Build history of the part. All positions in model axes, mm. A direction names the side the tool comes from. Coordinates: 2 decimals unless noted, no trailing zeros. Order: outer loops, then holes, each group sorted by start corner. A loop starts at its lowest first (then second) coordinate and runs counter-clockwise, first axis right, second up. Notation, with made-up numbers: M 12,-8 L 60,-8 A32 ccw 60,29 Z; hole C 24.25,49.5 d9. An arc over 180 degrees is marked long. Use a Markdown table: item, result. Add a question column.
from build123d import *

# Parameters (mm, degrees)
ESQUISSE1_W      = 187
ESQUISSE1_H      = 15
ESQUISSE1_R      = 1.5
EXTRUSION1_DEPTH = 1.5
ESQUISSE3_W      = 187
ESQUISSE3_H      = 1.5
EXTRUSION3_DEPTH = 13.5
ESQUISSE4_R      = 1.5
EXTRUSION4_DEPTH = 10


with BuildPart() as part:
    # Esquisse1 → Extrusion1 (new body)
    with BuildSketch(Plane.XY):
        with Locations((13.570945199, 9.544736842)):
            Rectangle(ESQUISSE1_W, ESQUISSE1_H)
        with Locations((101.070945199, 9.544736842)):
            Circle(ESQUISSE1_R, mode=Mode.SUBTRACT)
        with Locations((-72.429054801, 8.044736842)):
            Circle(ESQUISSE1_R, mode=Mode.SUBTRACT)
        with Locations((-31.429054801, 8.044736842)):
            Circle(ESQUISSE1_R, mode=Mode.SUBTRACT)
        with Locations((68.570945199, 8.044736842)):
            Circle(ESQUISSE1_R, mode=Mode.SUBTRACT)
    extrude(amount=EXTRUSION1_DEPTH)

    # Esquisse3 → Extrusion3 (add)
    with BuildSketch(Plane.XY.offset(1.5)):
        with Locations((13.570945199, 16.294736842)):
            Rectangle(ESQUISSE3_W, ESQUISSE3_H)
    extrude(amount=EXTRUSION3_DEPTH)

    # Esquisse4 → Extrusion4 (cut)
    with BuildSketch(Plane.XZ.offset(-15.544736842)):
        with Locations((-72.429054801, 7.5)):
            Circle(ESQUISSE4_R)
    extrude(amount=-EXTRUSION4_DEPTH, mode=Mode.SUBTRACT)


solid = part.part
(1) Slice it at C-C on y = 13.75. Give the cut face in (x, z), and give its area (4 significant figures).
(2) Drill centre lines: line 1 along Y through (x, z) = (65, 11.25); line 2 along Z through (x, y) = (56, 10); line 3 along Y through (x, z) = (68, 0.5). Where is each one in solid material? Low to high. Write a range as from..to.
(3) Drop flat-ended pins along their axis: P1, Ø5, axis at x = 31, y = 6.5, coming from the +Z side; P2, Ø8, axis at x = 6.5, y = 12.5, coming from the +Z side; P3, Ø3.5, axis at x = -72.43, z = 7.5, coming from the -Y side. Give the stop position or say it passes through.
(4) Slice it at A-A on x = -35.5. Give the cut face in (y, z).
(5) Which spindle directions (+Z, -Z, +X, -X, +Y, -Y) get a long thin tool onto all of the face, cutting with end or side? Do faces 1 (the cylindrical face through (99.572, 9.611, 0.74)), 2 (the flat face through (12, 15.545, 8)). Say none if no direction does.
(6) Slice it at B-B on z = 3.5. Give the cut face in (x, y), and give its area (4 significant figures).
(7) Mould opens along X. For faces 3 (the flat face through (12, 9, 1.5)), 4 (the cylindrical face through (-73.928, 8.111, 0.74)), 5 (the flat face through (-79.929, 12, 1)) say: released by +X, released by -X, zero draft, split by the parting line, or undercut.
Solutions:
| question | item | result |
|---|---|---|
| 1 | outline | M -79.93,0 L 107.07,0 L 107.07,1.5 L -79.93,1.5 Z |
| 1 | area | 280.5 mm² |
| 2 | line 1 | 15.54..17.04 |
| 2 | line 2 | 0..1.5 |
| 2 | line 3 | 2.04..6.66, 9.43..17.04 |
| 3 | P1 | z = 1.5 |
| 3 | P2 | z = 15 |
| 3 | P3 | y = 15.54 |
| 4 | outline | M 2.04,0 L 17.04,0 L 17.04,15 L 15.54,15 L 15.54,1.5 L 2.04,1.5 Z |
| 5 | face 1 | +Z, -Z |
| 5 | face 2 | +Z, +X, -X, -Y |
| 6 | outline | M -79.93,15.54 L 107.07,15.54 L 107.07,17.04 L -79.93,17.04 Z |
| 6 | area | 280.5 mm² |
| 7 | face 3 | zero draft |
| 7 | face 4 | undercut |
| 7 | face 5 | released by -X |
